Verification items for the finished model (mm, model axes). Coordinates: 2 decimals unless noted, no trailing zeros. Order: outer loops, then holes, each group sorted by start corner. A loop starts at its lowest first (then second) coordinate and runs counter-clockwise, first axis right, second up. Notation, with made-up numbers: M 6,29.5 L 26,29.5 A28 cw 26,47.5 Z; hole C -14.75,1.25 d4. An arc over 180 degrees is marked long. Return JSON: item names as keys, results as strings. Group by question number.
Q1. Section check C-C, the plane x = -12.75. Enter the section's corners in (y, z), then the cut area to 3 significant figures.
Q2. Go/stop test with a flat-tipped pin: pin 1 Ø4 at (x, y) = (-44.25, 54.22) entering from -Z. Record where the tip stops, or that it passes through.
Q3. Section check A-A, the plane x = -31. Enter the section's corners in (y, z).
Q4. Thickness scan on probe 1 along Y at (x, z) = (-12.75, 0.45); probe 2 along X at (y, z) = (55, 0.1); probe 3 along Y at (x, z) = (-44.25, 0.55). Record the ranges inside material, lowest first.
Q5. Section check B-B, the plane y = 18.5. Enter the section's corners in (x, z).
Q6. Section check D-D, the plane z = 0.45. Enter the section's corners in (x, y).
from build123d import *

# Parameters (mm, degrees)
F0_R     = 2.5
F1_DEPTH = 1.6


with BuildPart() as f1:
    # F0 (on Top) → F1 (new body)
    with BuildSketch(Plane.XY):
        with BuildLine():
            Line((-44.25, 0), (0, 0))
            Line((0, 0), (0, 63))
            Line((0, 63), (-57, 63))
            Line((-57, 63), (-57, 9))
            Line((-57, 9), (-46.75, 9))
            ThreePointArc((-46.75, 9), (-44.25, 11.5), (-41.75, 9))
            ThreePointArc((-41.75, 9), (-42.482233047, 7.232233047), (-44.25, 6.5))
            Line((-44.25, 6.5), (-44.25, 0))
        make_face()
        with Locations((-12.75, 9.2245186158)):
            Circle(F0_R, mode=Mode.SUBTRACT)
        with BuildLine():
            ThreePointArc((-46.75, 54.2245186158), (-44.25, 56.7245186158), (-41.75, 54.2245186158))
            ThreePointArc((-41.75, 54.2245186158), (-44.25, 51.7245186158), (-46.75, 54.2245186158))
        make_face(mode=Mode.SUBTRACT)
        with BuildLine():
            ThreePointArc((-8.5, 31.7245186158), (-42.6421356237, 17.582382992), (-28.5, 51.7245186158))
            ThreePointArc((-28.5, 51.7245186158), (-14.3578643763, 45.8666542395), (-8.5, 31.7245186158))
        make_face(mode=Mode.SUBTRACT)
        with BuildLine():
            ThreePointArc((-15.25, 54.2245186158), (-12.75, 56.7245186158), (-10.25, 54.2245186158))
            ThreePointArc((-10.25, 54.2245186158), (-12.75, 51.7245186158), (-15.25, 54.2245186158))
        make_face(mode=Mode.SUBTRACT)
        with BuildLine():
            Line((-57, 0), (-44.25, 0))
            Line((-44.25, 0), (-44.25, 6.5))
            ThreePointArc((-44.25, 6.5), (-46.017766953, 7.232233047), (-46.75, 9))
            Line((-46.75, 9), (-57, 9))
            Line((-57, 9), (-57, 0))
        make_face()
    extrude(amount=F1_DEPTH)


solid = f1.part
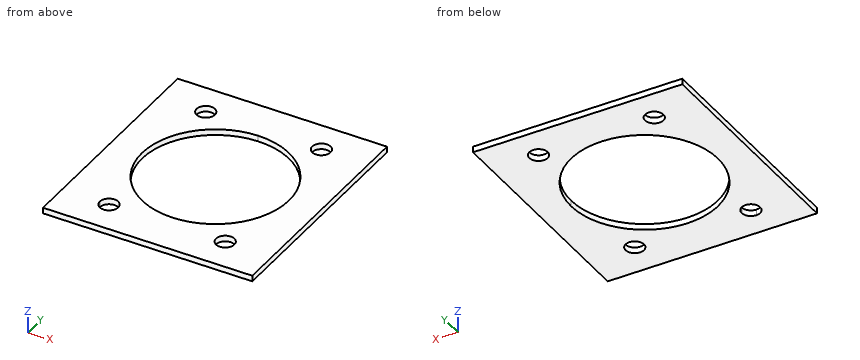
Numbers:
{
 "1": {"outline": "M 0,0 L 6.72,0 L 6.72,1.6 L 0,1.6 Z; M 11.72,0 L 19.4,0 L 19.4,1.6 L 11.72,1.6 Z; M 44.05,0 L 51.72,0 L 51.72,1.6 L 44.05,1.6 Z; M 56.72,0 L 63,0 L 63,1.6 L 56.72,1.6 Z", "area": "45.4 mm2"},
 "2": {"pin 1": "passes through"},
 "3": {"outline": "M 0,0 L 11.88,0 L 11.88,1.6 L 0,1.6 Z; M 51.57,0 L 63,0 L 63,1.6 L 51.57,1.6 Z"},
 "4": {"probe 1": "y = 0 to 6.72, 11.72 to 19.4, 44.05 to 51.72, 56.72 to 63", "probe 2": "x = -57 to -46.63, -41.87 to -15.13, -10.37 to 0", "probe 3": "y = 0 to 6.5, 11.5 to 19.4, 44.05 to 51.72, 56.72 to 63"},
 "5": {"outline": "M -57,0 L -43.5,0 L -43.5,1.6 L -57,1.6 Z; M -13.5,0 L 0,0 L 0,1.6 L -13.5,1.6 Z"},
 "6": {"outline": "M -57,0 L 0,0 L 0,63 L -57,63 Z; hole C -28.5,31.72 d40; hole C -44.25,9 d5; hole C -44.25,54.22 d5; hole C -12.75,9.22 d5; hole C -12.75,54.22 d5"}
}
